from build123d import *

# Parameters (mm, degrees)
SKETCH_W             = 80
SKETCH_H             = 40
PAD_DEPTH            = 50
SKETCH002_R          = 4.5
POCKET_DEPTH         = 50.001
SKETCH015_R          = 8.5
POCKET001_DEPTH      = 25
SKETCH004_W          = 70
SKETCH004_H          = 57
POCKET002_DEPTH      = 15
POCKET002_DEPTH_BACK = 100
SKETCH005_R          = 1.4
SKETCH005_W          = 58
SKETCH005_H          = 11.5
POCKET003_DEPTH      = 5
SKETCH006_W          = 3.5
SKETCH006_H          = 7
POCKET004_DEPTH      = 80.001
SKETCH007_W          = 10
SKETCH007_H          = 8
POCKET005_DEPTH      = 10
PAD002_DEPTH         = 29
SKETCH009_R          = 4.5
POCKET006_DEPTH      = 50.001
SKETCH013_W          = 9
SKETCH013_H          = 5.749281
POCKET007_DEPTH      = 5
POCKET007_DEPTH_BACK = 100
SKETCH014_W          = 11.905407
SKETCH014_H          = 10.178417
PAD003_DEPTH         = 0.3
POCKET029_DEPTH      = 95.001
SKETCH018_R          = 1.4
POCKET030_DEPTH      = 9
SKETCH019_R          = 2.4
POCKET031_DEPTH      = 10
POCKET032_DEPTH      = 50.001
SKETCH021_W          = 4
SKETCH021_H          = 8
POCKET033_DEPTH      = 28.001
SKETCH025_R          = 2.75
PAD014_DEPTH         = 6
SKETCH049_R          = 1.4
POCKET039_DEPTH      = 6
SKETCH044_R          = 5
POCKET040_DEPTH      = 35
PAD015_DEPTH         = 31
POCKET041_DEPTH      = 40
CHAMFER015_SIZE      = 1
CHAMFER016_SIZE      = 1
CHAMFER017_SIZE      = 1
CHAMFER018_SIZE      = 1


with BuildPart() as part:
    # Sketch → Pad (new body)
    with BuildSketch(Plane.XY):
        with Locations((0, 20)):
            Rectangle(SKETCH_W, SKETCH_H)
    extrude(amount=PAD_DEPTH)

    # Sketch002 → Pocket (cut, through all)
    with BuildSketch(Plane.XY.offset(50)):
        with Locations((10, 10)):
            Circle(SKETCH002_R)
    extrude(amount=-POCKET_DEPTH, mode=Mode.SUBTRACT)

    # Sketch015 (on Face5 of Pocket) → Pocket001 (cut)
    with BuildSketch(Plane.XY.offset(50)):
        with Locations((10, 10)):
            Circle(SKETCH015_R)
    extrude(amount=-POCKET001_DEPTH, mode=Mode.SUBTRACT)

    # Sketch004 → Pocket002 (cut, two sides)
    with BuildSketch(Plane(origin=(0, 35, 0), x_dir=(-1, 0, 0), z_dir=(0, 1, 0))) as pocket002_sk:
        with Locations((0, 31.5)):
            Rectangle(SKETCH004_W, SKETCH004_H)
    extrude(amount=-POCKET002_DEPTH, mode=Mode.SUBTRACT)
    extrude(pocket002_sk.sketch, amount=POCKET002_DEPTH_BACK, mode=Mode.SUBTRACT)

    # Sketch005 → Pocket003 (cut)
    with BuildSketch(Plane.XY.offset(3)):
        with Locations((-31.75, 31)):
            Circle(SKETCH005_R)
        with Locations((31.75, 31)):
            Circle(SKETCH005_R)
        with Locations((0, 31)):
            Rectangle(SKETCH005_W, SKETCH005_H)
    extrude(amount=-POCKET003_DEPTH, mode=Mode.SUBTRACT)

    # Sketch006 → Pocket004 (cut, through all)
    with BuildSketch(Plane(origin=(-40, 0, 0), x_dir=(0, -1, 0), z_dir=(-1, 0, 0))):
        with Locations((-11.75, 13.5)):
            Rectangle(SKETCH006_W, SKETCH006_H)
    extrude(amount=-POCKET004_DEPTH, mode=Mode.SUBTRACT)

    # Sketch007 → Pocket005 (cut)
    with BuildSketch(Plane(origin=(0, 20, 0), x_dir=(-1, 0, 0), z_dir=(0, 1, 0))):
        with Locations((-30, 14)):
            Rectangle(SKETCH007_W, SKETCH007_H)
        with Locations((30, 14)):
            Rectangle(SKETCH007_W, SKETCH007_H)
    extrude(amount=-POCKET005_DEPTH, mode=Mode.SUBTRACT)

    # Sketch008 → Pad002 (join)
    with BuildSketch(Plane(origin=(0, 35, 0), x_dir=(-1, 0, 0), z_dir=(0, 1, 0))):
        Polygon((40, 29), (55, 44), (55, 50), (40, 50), align=None)
    extrude(amount=-PAD002_DEPTH)

    # Sketch009 → Pocket006 (cut, through all)
    with BuildSketch(Plane.XY.offset(50)):
        with Locations((-47, 20)):
            Circle(SKETCH009_R)
    extrude(amount=-POCKET006_DEPTH, mode=Mode.SUBTRACT)

    # Sketch013 → Pocket007 (cut, two sides)
    with BuildSketch(Plane(origin=(-52, 0, 0), x_dir=(0, -1, 0), z_dir=(-1, 0, 0))) as pocket007_sk:
        with Locations((-20, 39.025359)):
            Rectangle(SKETCH013_W, SKETCH013_H)
    extrude(amount=-POCKET007_DEPTH, mode=Mode.SUBTRACT)
    extrude(pocket007_sk.sketch, amount=POCKET007_DEPTH_BACK, mode=Mode.SUBTRACT)

    # Sketch014 → Pad003 (join)
    with BuildSketch(Plane(origin=(0, 0, 41.900547), x_dir=(1, 0, 0), z_dir=(0, 0, -1))):
        with Locations((-46.607828, -20.201936)):
            Rectangle(SKETCH014_W, SKETCH014_H)
    extrude(amount=-PAD003_DEPTH)

    # Sketch017 → Pocket029 (cut, through all)
    with BuildSketch(Plane.YZ.offset(40)):
        Polygon((4, 53.2), (4, 30), (1.5, 30), (1.5, 20), (-2.11, 20), (-2.11, 61.28), align=None)
    extrude(amount=-POCKET029_DEPTH, mode=Mode.SUBTRACT)

    # Sketch018 → Pocket030 (cut)
    with BuildSketch(Plane.XY.offset(50)):
        with Locations((-35, 12)):
            Circle(SKETCH018_R)
        with Locations((35, 12)):
            Circle(SKETCH018_R)
    extrude(amount=-POCKET030_DEPTH, mode=Mode.SUBTRACT)

    # Sketch019 → Pocket031 (cut)
    with BuildSketch(Plane(origin=(0, 0, 0), x_dir=(1, 0, 0), z_dir=(0, 0, -1))):
        with Locations((-30, -5)):
            Circle(SKETCH019_R)
        with Locations((30, -5)):
            Circle(SKETCH019_R)
    extrude(amount=-POCKET031_DEPTH, mode=Mode.SUBTRACT)

    # Sketch020 → Pocket032 (cut, through all)
    with BuildSketch(Plane(origin=(0, 0, 0), x_dir=(1, 0, 0), z_dir=(0, 0, -1))):
        with BuildLine():
            ThreePointArc((15.5, -10), (10, -4.5), (4.5, -10))
            Line((4.5, -10), (-0.5, -10))
            Line((-0.5, -10), (-0.5, 2.44))
            Line((-0.5, 2.44), (20.5, 2.44))
            Line((20.5, -10), (20.5, 2.44))
            Line((15.5, -10), (20.5, -10))
        make_face()
    extrude(amount=-POCKET032_DEPTH, mode=Mode.SUBTRACT)

    # Sketch021 → Pocket033 (cut, through all)
    with BuildSketch(Plane.XZ.offset(-12)):
        with Locations((18, 14)):
            Rectangle(SKETCH021_W, SKETCH021_H)
        with Locations((2, 14)):
            Rectangle(SKETCH021_W, SKETCH021_H)
    extrude(amount=-POCKET033_DEPTH, mode=Mode.SUBTRACT)

    # Sketch025 (on Face1 of Pocket033) → Pad014 (join)
    with BuildSketch(Plane(origin=(0, 40, 0), x_dir=(-1, 0, 0), z_dir=(0, 1, 0))):
        with Locations((-36, 3.5)):
            Circle(SKETCH025_R)
    pad014 = extrude(amount=-PAD014_DEPTH)

    # Mirrored002: Pad014 across Sketch025 V_Axis
    add(pad014.mirror(Plane(origin=(0, 40, 0), x_dir=(0, 1, 0), z_dir=(-1, 0, 0))))

    # Sketch049 (on Face1 of Mirrored002) → Pocket039 (cut)
    with BuildSketch(Plane(origin=(0, 40, 0), x_dir=(-1, 0, 0), z_dir=(0, 1, 0))):
        with Locations((-36, 3.5)):
            Circle(SKETCH049_R)
    pocket039 = extrude(amount=-POCKET039_DEPTH, mode=Mode.SUBTRACT)

    # Mirrored003: Pocket039 across Sketch049 V_Axis
    add(pocket039.mirror(Plane(origin=(0, 40, 0), x_dir=(0, 1, 0), z_dir=(-1, 0, 0))), mode=Mode.SUBTRACT)

    # Sketch044 → Pocket040 (cut)
    with BuildSketch(Plane.XY.offset(50)):
        with Locations((-31, 23)):
            Circle(SKETCH044_R)
    extrude(amount=-POCKET040_DEPTH, mode=Mode.SUBTRACT)

    # Sketch026 → Pad015 (join)
    with BuildSketch(Plane.XY.offset(50)):
        with BuildLine():
            ThreePointArc((21.221659, 13.061419), (12.186737, 21.372713), (0.660759, 17.14669))
            Line((1.758582, 14.664218), (0.660759, 17.14669))
            ThreePointArc((19.018099, 12.326896), (11.159892, 19.192932), (1.758582, 14.664218))
            Line((19.018099, 12.326896), (21.221659, 13.061419))
        make_face()
    extrude(amount=-PAD015_DEPTH)

    # Sketch042 → Pocket041 (cut)
    with BuildSketch(Plane.YZ.offset(40)):
        Polygon((26, 10.194524), (33.8, 14.697856), (33.8, 23.70452), (26, 28.207852), (18.2, 23.70452), (18.2, 14.697856), align=None)
        Polygon((31.6, 39.037417), (31.6, 43.194339), (28, 45.2728), (24.4, 43.194339), (24.4, 39.037417), (28, 36.958956), align=None)
    extrude(amount=-POCKET041_DEPTH, mode=Mode.SUBTRACT)

    # Chamfer015
    chamfer015_edges = [part.edges().sort_by_distance(p)[0] for p in [
        (40, 20, 0),
        (-40, 20, 0),
    ]]
    chamfer(chamfer015_edges, length=CHAMFER015_SIZE)

    # Chamfer016
    chamfer016_edges = [part.edges().sort_by_distance(p)[0] for p in [
        (-55, 35, 47),
        (-55, 6, 47),
        (-47.5, 6, 36.5),
    ]]
    chamfer(chamfer016_edges, length=CHAMFER016_SIZE)

    # Chamfer017
    chamfer017_edges = [part.edges().sort_by_distance(p)[0] for p in [
        (-0.5, 4, 40),
        (20.5, 4, 40),
        (20.5, 1.5, 25),
        (-0.5, 1.5, 25),
        (-0.5, 0, 10),
        (20.5, 0, 10),
    ]]
    chamfer(chamfer017_edges, length=CHAMFER017_SIZE)

    # Chamfer018
    chamfer018_edges = [part.edges().sort_by_distance(p)[0] for p in [
        (40, 0, 10.5),
        (40, 1.5, 25),
        (40, 4, 40),
        (-40, 0, 10.5),
        (-40, 1.5, 25),
        (-40, 4, 40),
    ]]
    chamfer(chamfer018_edges, length=CHAMFER018_SIZE)


solid = part.part
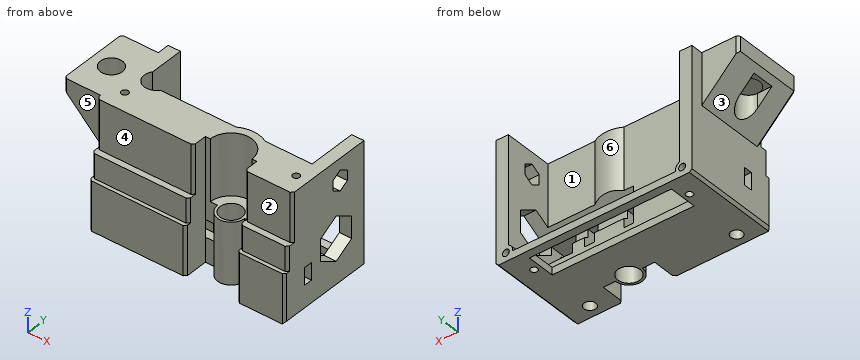
Can you work these out from the model? Positions are in its coordinate system, mm. Face numbers are marked on the shaded views. A direction names the side the tool comes from. Coordinates: 2 decimals unless noted, no trailing zeros. Write each loop counter-clockwise with the first axis right and the second up, starting at its lowest first coordinate (ties: lowest second). Pieces come first, ordered by that corner, then holes. Notation, with made-up numbers: (-29.5, -22.75) - (22.5, -22.75) arc R19 cw to (22.5, 7.25) - close; hole circle Ø11 at (-32.75, 70.5). An arc over 180 degrees is marked (long way). Return JSON: item names as keys, results as strings. Group by question number.
Item 1: I'm going to push flat-ended pins straight in: pin 1 Ø1.4 at (x, y) = (-30, 5.5) entering from -Z; pin 2 Ø0.8 at (x, y) = (-13, 1) entering from +Z; pin 3 Ø16 at (x, y) = (3.5, 30) entering from +Z. Where does each tip first touch, or does it pass through?
Item 2: Please list where these lines run through material, in increasing order: probe 1 along X at (y, z) = (37.5, 3.5); probe 2 along X at (y, z) = (15, 13.5); probe 3 along Z at (x, y) = (36, 35.25).
Item 3: If we section it at B-B (z = 47): Count the separate pieces of the cut face and the enclosed holes in it, then the cut area to 3 significant figures.
Item 4: We'd pull the mould along X, two halves only. Please class the marked faces 1, 2 and 3: pulls with the +X half, pulls with the -X half, needs draft (parallel to the pull), parting line crosses it, or undercut.
Item 5: Which directions (+Z, -Z, +X, -X, +Y, -Y) give clear straight access to the entire face, cutting with the end or side of a thin tool? Please do the marked faces 4, 5 and 6.
Item 6: If we section it at A-A (z = 19): Write out the boundary of the cut face in (x, y).
Item 7: If we section it at C-C (x = 11.5): Write out the boundary of the cut face in (y, z).
Return value:
{
 "1": {"pin 1": "stops at z = 10", "pin 2": "stops at z = 20", "pin 3": "stops at z = 3"},
 "2": {"probe 1": "x = -40 to -37.4, -34.6 to -33.25, 33.25 to 34.6, 37.4 to 40", "probe 2": "x = -40 to -35, -25 to 0, 4 to 16, 20 to 25, 35 to 40", "probe 3": "z = 0 to 2.1, 4.9 to 50"},
 "3": {"separate pieces": "1", "enclosed holes": "3", "area": "1,590 mm^2"},
 "4": {"face 1": "undercut", "face 2": "needs draft", "face 3": "pulls with the -X half"},
 "5": {"face 4": "+Z, +X, -X, -Y", "face 5": "+Z, -Z, -X, -Y", "face 6": "+Z, +Y"},
 "6": {"outline": "(-40, 1) - (-39, 0) - (-1.5, 0) - (-0.5, 1) - (-0.5, 10) - (4.5, 10) arc R5.5 ccw to (15.5, 10) - (20.5, 10) - (20.5, 1) - (21.5, 0) - (39, 0) - (40, 1) - (40, 18.2) - (0, 18.2) - (0, 20) - (-27, 20) arc R5 cw to (-35, 26) - (-35, 40) - (-40, 40) - close; (35, 33.8) - (40, 33.8) - (40, 40) - (35, 40) - close; hole circle Ø9 at (10, 10)"},
 "7": {"outline": "(4.71, 0) - (5.76, 0) - (5.76, 25) - (4.71, 25) - close; (14.24, 0) - (25.25, 0) - (25.25, 3) - (20, 3) - (20, 13.66) - (18.2, 14.7) - (18.2, 23.7) - (21.49, 25.6) - (21.49, 50) - (18.37, 50) - (18.37, 25) - (14.24, 25) - close; (36.75, 0) - (40, 0) - (40, 3) - (36.75, 3) - close"}
}
